Autodesk Fusion 360 part; units mm, degrees
sketch "Skizze1" plane through (0, 0, 0) normal (0, 0, 1) x (1, 0, 0)
  line L0 (-3, 0) -> (-3, 0.8)
  line L1 (-3, 0.8) -> (-2.5, 0.8)
  line L2 (-2.5, 0.8) -> (-2.5, 2.1)
  line L3 (-8.4843, 2.1) -> (11.6981, 2.1) construction
  line L4 (0, 9) -> (0, -6.2163) construction
  arc A0 (0, 4.6) -> (-2.5, 2.1) centre (0, 2.1) ccw
  line L5 (0, 4.6) -> (0, 0)
  line L6 (0, 0) -> (-3, 0)
  line L7 (2.5, 2) -> (4.5, 2)
  line L8 (4.5, 2) -> (4.5, -2)
  line L9 (4.5, -2) -> (2.5, -2)
  line L10 (2.5, -2) -> (2.5, 2)
  line L11 (-4.5, 2) -> (-2.5, 2)
  line L12 (-2.5, 2) -> (-2.5, -2)
  line L13 (-2.5, -2) -> (-4.5, -2)
  line L14 (-4.5, -2) -> (-4.5, 2)
  point P0 (0, 2.1)
  dimension "d1" = 3
  dimension "d2" = 0.8
  dimension "d3" = 2.5
  dimension "d7" = 2.5
  dimension "d8" = 2
  dimension "d9" = 2
  dimension "d10" = 2
  dimension "d117" = 2.5
  dimension "d119" = 2
  dimension "d120" = 2
  dimension "d121" = 2
  dimension "d122" = 2.1
  dimension "d123" = 4.6
revolve "Drehen1" add sketch "Skizze1" angle 360 about axis through (0, 9, 0) along (0, -1, 0) contours L0 L1 L6 L12 | L2 A0 L5 L6 L12 makes body 1
sketch "Skizze2" plane through (0, 0, 0) normal (0, 0, 1) x (1, 0, 0)
  line L0 (-10, 20) -> (10, 20)
  line L1 (10, 20) -> (10, -6.2)
  line L2 (10, -6.2) -> (-10, -6.2)
  line L3 (-10, -6.2) -> (-10, 20)
  line L4 (0, 21.3723) -> (0, -17) construction
  line L5 (-26.2349, 0) -> (38.3962, 0) construction
  line L6 (5, -6.2) -> (5, 3.8)
  line L7 (5, 3.8) -> (10, 3.8)
  line L8 (-5, -6.2) -> (-5, 3.8)
  line L9 (-5, 3.8) -> (-10, 3.8)
  line L10 (-17, 10) -> (24.4562, 10) construction
  line L11 (-5, 26) -> (-5, 5) construction
  line L12 (5, 25.6741) -> (5, 5) construction
  circle A0 centre (-5, 10) radius 1.75
  circle A1 centre (5, 10) radius 1.75
  line L13 (-16, 15) -> (36.57, 15) construction
  circle A2 centre (0, 15) radius 1.75
  line L14 (-7, 22.2425) -> (-7, -4.6464) construction
  line L15 (7, 22.2425) -> (7, -3.3633) construction
  circle A3 centre (-7, 15) radius 2
  circle A4 centre (7, 15) radius 2
  dimension "d13" = 10
  dimension "d14" = 10
  dimension "d15" = 6.2
  dimension "d16" = 20
  dimension "d32" = 5
  dimension "d33" = 10
  dimension "d34" = 5
  dimension "d35" = 10
  dimension "d36" = 10
  dimension "d37" = 5
  dimension "d38" = 5
  dimension "d39" = 3.5
  dimension "d40" = 3.5
  dimension "d41" = 5
  dimension "d42" = 3.5
  dimension "d53" = 7
  dimension "d54" = 7
extrude "Extrusion2" add sketch "Skizze2" against normal blind 10 separate body contours L0 L1 L2 L3 L6 L7 L8 L9 | A3 | A4 makes body 2
extrude "Extrusion7" cut sketch "Skizze2" against normal blind 5 contours A3 | A4 bodies 2
combine "Kombinieren1" operation cut target body 2 tool bodies 1
sketch "Skizze4" plane through (0, 0, 0) normal (0, 0, 1) x (1, 0, 0)
  line L0 (2.15, -6.2) -> (-2.15, -6.2)
  line L1 (-2.15, -6.2) -> (-2.15, 0)
  line L2 (-2.15, 0) -> (2.15, 0)
  line L3 (2.15, 0) -> (2.15, -6.2)
  line L4 (2.15, -6.2) -> (-2.15, 0) construction
  line L5 (-2.15, -6.2) -> (2.15, 0) construction
  line L6 (0, 9.7025) -> (0, -8.7035) construction
  line L7 (-7.2352, -6.2) -> (6.1757, -6.2) construction
  point P0 (0, -3.1)
  point P1 (0, -6.2)
  dimension "d21" = 4.3
  dimension "d22" = 6.2
extrude "Extrusion4" cut sketch "Skizze4" against normal blind 0.25 bodies 2
ref_plane "Arbeitsebene1" through (0, 0, -6.5) normal (0, 0, 1) x (1, 0, 0)
sketch "Skizze7" plane through (0, 0, -6.5) normal (0, 0, 1) x (1, 0, 0)
  line L0 (-16.0259, 10) -> (20, 10) construction
  line L1 (-5, 21.68) -> (-5, -11.619) construction
  line L2 (5, 22.2413) -> (5, -12.5543) construction
  line L3 (-2.05, 11.7032) -> (-5, 13.4064)
  line L4 (-5, 13.4064) -> (-7.95, 11.7032)
  line L5 (-7.95, 11.7032) -> (-7.95, 8.2968)
  line L6 (-7.95, 8.2968) -> (-5, 6.5936)
  line L7 (-5, 6.5936) -> (-2.05, 8.2968)
  line L8 (-2.05, 8.2968) -> (-2.05, 11.7032)
  line L9 (7.95, 11.7032) -> (5, 13.4064)
  line L10 (5, 13.4064) -> (2.05, 11.7032)
  line L11 (2.05, 11.7032) -> (2.05, 8.2968)
  line L12 (2.05, 8.2968) -> (5, 6.5936)
  line L13 (5, 6.5936) -> (7.95, 8.2968)
  line L14 (7.95, 8.2968) -> (7.95, 11.7032)
  line L15 (-15.7752, 15) -> (18.7006, 15) construction
  line L16 (0, 22.633) -> (0, -9.7229) construction
  line L17 (2.95, 16.7032) -> (0, 18.4064)
  line L18 (0, 18.4064) -> (-2.95, 16.7032)
  line L19 (-2.95, 16.7032) -> (-2.95, 13.2968)
  line L20 (-2.95, 13.2968) -> (0, 11.5936)
  line L21 (0, 11.5936) -> (2.95, 13.2968)
  line L22 (2.95, 13.2968) -> (2.95, 16.7032)
  point P0 (-5, 10)
  point P1 (5, 10)
  point P2 (-5, 10)
  point P3 (5, 10)
  point P4 (0, 15)
  point P5 (0, 15)
  dimension "d44" = 10
  dimension "d45" = 5
  dimension "d46" = 5
  dimension "d47" = 5.9
  dimension "d48" = 5.9
  dimension "d51" = 15
  dimension "d52" = 5.9
extrude "Extrusion6" cut sketch "Skizze7" along normal blind 2.8 bodies 2
equation "d3 = Linear Dimension-4"
equation "d7 = Linear Dimension-7"
equation "d117 = Linear Dimension-11"
equation "d122 = 4.6 mm - d"
Read the model definition and answer for the solid it produces. Units are mm, in the model's axes. A direction names the side the tool comes from. Give positions to 0.01 mm unless a question says otherwise; leave off trailing zeros. Order: outer loops, then holes, each group sorted by start corner. A loop starts at its lowest first (then second) coordinate and runs counter-clockwise, first axis right, second up. Notation, with made-up numbers: (81, 14) -> (139, 14) arc R12 cw to (139, 29) -> close; hole circle Ø8 at (26, 38.5). An arc over 180 degrees is marked (long way). Write item = value, one per line.
1. Given pin 1 (2.5 mm diameter, centred on x = 8, z = -7, fed in from -Y); pin 2 (3 mm diameter, centred on x = -6.5, y = 9, fed in from +Z); pin 3 (2 mm diameter, centred on x = -7, y = 15.5, fed in from +Z); pin 4 (3 mm diameter, centred on x = 0, y = 15, fed in from +Z), each flat-ended and moving along its own axis, determine where each tip first touches the part or whether it passes through.
Numbers:
pin_1 = 3.8
pin_2 = 0
pin_3 = -5
pin_4 = through
2. A cutting plane is placed at D-D, the plane y = 10. Write down the section's boundary in (x, z).
Numbers:
outline = (-10, -10) -> (-6.75, -10) -> (-6.75, -6.5) -> (-7.95, -6.5) -> (-7.95, -3.7) -> (-6.75, -3.7) -> (-6.75, 0) -> (-10, 0) -> close; (-3.25, -10) -> (3.25, -10) -> (3.25, -6.5) -> (2.05, -6.5) -> (2.05, -3.7) -> (3.25, -3.7) -> (3.25, 0) -> (-3.25, 0) -> (-3.25, -3.7) -> (-2.05, -3.7) -> (-2.05, -6.5) -> (-3.25, -6.5) -> close; (6.75, -10) -> (10, -10) -> (10, 0) -> (6.75, 0) -> (6.75, -3.7) -> (7.95, -3.7) -> (7.95, -6.5) -> (6.75, -6.5) -> close
3. Straight lines are drawn through the part: line 1 along Y through (x, z) = (0, -2.6); line 2 along X through (y, z) = (16.25, -0.75); line 3 along Y through (x, z) = (0, -9.1). For each, find the intervals that lie inside material, in ascending order.
Numbers:
line_1 = -6.2 to 0, 0.8 to 13.25, 16.75 to 20
line_2 = -10 to -8.56, -5.44 to -1.22, 1.22 to 5.44, 8.56 to 10
line_3 = -6.2 to 13.25, 16.75 to 20
4. For faces 4 (the face through (5, -1, -5)), 5 (the face through (-2.05, 10, -5)), 6 (the face through (3.71, 11.18, -1.82)), 7 (the face through (-5, -1, -5)), 8 (the face through (0, 0, -2)), determine the directions among +Z, -Z, +X, -X, +Y, -Y from which every point of the face is accessible in a straight line to the end or side of a thin tool.
Numbers:
face_4 = +Z, -Z, +X, -Y
face_5 = none
face_6 = +Z, -Z
face_7 = +Z, -Z, -X, -Y
face_8 = +Z
5. A cutting plane is placed at C-C, the plane x = 0.5. Write down the section's boundary in (y, z), and give its area (3 significant figures).
Numbers:
outline = (-6.2, -10) -> (13.32, -10) -> (13.32, -6.5) -> (11.88, -6.5) -> (11.88, -3.7) -> (13.32, -3.7) -> (13.32, 0) -> (4.55, 0) arc R2.45 cw to (2.1, -2.45) -> (0.8, -2.45) -> (0.8, -2.96) -> (0, -2.96) -> (0, -0.25) -> (-6.2, -0.25) -> close; (16.68, -10) -> (20, -10) -> (20, 0) -> (16.68, 0) -> (16.68, -3.7) -> (18.12, -3.7) -> (18.12, -6.5) -> (16.68, -6.5) -> close
area = 209 mm²
6. A cutting plane is placed at B-B, the plane z = -7.25. Write down the section's boundary in (x, y).
Numbers:
outline = (-10, 3.8) -> (-5, 3.8) -> (-5, -6.2) -> (5, -6.2) -> (5, 3.8) -> (10, 3.8) -> (10, 20) -> (-10, 20) -> close; hole circle Ø3.5 at (-5, 10); hole circle Ø3.5 at (0, 15); hole circle Ø3.5 at (5, 10)
7. The mould has two halves that part along Y. Classify faces 1 (the face through (-3.7, 8.5, -6.5)), 2 (the face through (10, 12, -5)), 3 (the face through (0, 20, -5)): +Y half, -Y half, draft (parallel to the pull), parting line (faces both ways), or undercut.
Numbers:
face_1 = undercut
face_2 = draft
face_3 = +Y half
8. A cutting plane is placed at A-A, the plane y = 15. Write down the section's boundary in (x, z).
Numbers:
outline = (-10, -10) -> (-1.75, -10) -> (-1.75, -6.5) -> (-2.95, -6.5) -> (-2.95, -3.7) -> (-1.75, -3.7) -> (-1.75, 0) -> (-5, 0) -> (-5, -5) -> (-9, -5) -> (-9, 0) -> (-10, 0) -> close; (1.75, -10) -> (10, -10) -> (10, 0) -> (9, 0) -> (9, -5) -> (5, -5) -> (5, 0) -> (1.75, 0) -> (1.75, -3.7) -> (2.95, -3.7) -> (2.95, -6.5) -> (1.75, -6.5) -> close
